Geometry: final body of the model. Coordinates: model frame, mm. A direction names the side the tool comes from. Coordinates: 2 decimals unless noted, no trailing zeros. Order: outer loops, then holes, each group sorted by start corner. A loop starts at its lowest first (then second) coordinate and runs counter-clockwise, first axis right, second up. Notation, with made-up numbers: (34, -12.5) -> (72, -12.5) arc R19 cw to (72, 19.5) -> close; hole circle Ø2 at (1, 13). An arc over 180 degrees is marked (long way). Answer in a Markdown table with one row per item. Add a question column.
1) Ray query, line 1 (Y direction, x = -2.75, z = 8); line 2 (Y direction, x = 8.25, z = 14.5); line 3 (Z direction, x = -5.75, y = 4). Return the intervals inside material, ascending. Write a range as from..to.
2) Set-up query: faces 1 (the face through (0, 2, 9.431)), 2 (the face through (-0.7, 2.1, 11.831)), 3 (the face through (6.972, 6.529, 14.967)), 4 (the face through (-2, 2, -5.169)). Return all of +Z, -Z, +X, -X, +Y, -Y with unobstructed straight access to the full face (end or side cutting, diameter ignored); none if empty.
3) Section query D-D on y = 1.5. Return the cut outline in (x, z).
4) Section query A-A on x = -5. Return the cut outline in (y, z), then the cut area to 3 significant figures.
5) Section query C-C on x = -2.5. Return the cut outline in (y, z), then the cut area to 3 significant figures.
6) Contact query for flat-ended pins moving along their axis: P1, Ø6, axis at x = -4, y = -1, coming from the -Z side; P2, Ø4, axis at y = -9.48, z = -8.17, coming from the -X side; P3, Ø3, axis at x = -6, y = 1, coming from the +Z side. Output: stop coordinate, or through.
7) Section query B-B on z = 9. Return the cut outline in (x, y), then the cut area to 3 significant figures.
8) Pull-direction query (X, two-part tool) for faces 5 (the face through (-2.29, 0.57, 10.65)), 6 (the face through (6.972, 13.65, -1.186)), 7 (the face through (-10, 9, 3)); classes: +X half, -X half, draft (parallel to the pull), parting line (faces both ways), or undercut.
Autodesk Fusion 360 part; units mm, degrees
sketch "Sketch2" plane through (5, 0, 0) normal (1, 0, 0) x (0, 1, 0)
  line L0 (16.9637, 18.2844) -> (-13.0292, -11.7227) construction
  line L1 (-12.9363, 18.2856) -> (17.0619, -11.7162) construction
  circle A0 centre (13.5169, 14.8306) radius 1.6
  circle A1 centre (-9.4831, 14.8306) radius 1.6
  circle A2 centre (-9.4831, -8.1694) radius 1.6
  circle A3 centre (13.5169, -8.1694) radius 1.6
  circle A4 centre (-9.4831, 14.8306) radius 4.1
  circle A5 centre (13.5169, 14.8306) radius 4.1
  circle A6 centre (-9.4831, -8.1694) radius 4.1
  line L2 (9.4619, 10.7862) -> (-5.5274, -4.2245) construction
  line L3 (-7.1431, 18.1972) -> (2.0169, 11.8306)
  line L4 (2.0169, 11.8306) -> (11.1769, 18.1972)
  line L5 (-12.8477, 12.4876) -> (-6.471, 3.3306)
  line L6 (-6.471, 3.3306) -> (-12.8477, -5.8265)
  line L7 (-7.1431, -11.5361) -> (2.0169, -5.1694)
  line L8 (10.5048, 3.3306) -> (16.8815, 12.4876)
  circle A7 centre (13.5169, -8.1694) radius 4.1
  line L9 (10.5048, 3.3306) -> (16.8815, -5.8265)
  line L10 (2.0169, -5.1694) -> (11.1769, -11.5361)
  line L11 (-4.0831, -2.7694) -> (8.1169, -2.7694)
  line L12 (8.1169, -2.7694) -> (8.1169, 9.4306)
  line L13 (8.1169, 9.4306) -> (-4.0831, 9.4306)
  line L14 (-4.0831, 9.4306) -> (-4.0831, -2.7694)
  line L15 (-4.0831, -2.7694) -> (8.1169, 9.4306) construction
  line L16 (8.1169, -2.7694) -> (-4.0831, 9.4306) construction
  line L17 (10.5048, 11.8306) -> (-6.471, 11.8306)
  line L18 (-6.471, 11.8306) -> (-6.471, -5.1694)
  line L19 (-6.471, -5.1694) -> (10.5048, -5.1694)
  line L20 (10.5048, -5.1694) -> (10.5048, 11.8306)
  line L21 (10.5048, 11.8306) -> (-6.471, -5.1694) construction
  line L22 (-6.471, 11.8306) -> (10.5048, -5.1694) construction
  point P0 (2.0169, 3.3306)
  point P1 (2.0169, 3.3306)
  point P2 (2.0169, 3.3306)
  point P3 (2.0169, 3.3306)
  point P4 (2.0169, 3.3306)
  dimension "d11" = 3.2
  dimension "d12" = 11.5
  dimension "d13" = 3.2
  dimension "d14" = 3.2
  dimension "d15" = 3.2
  dimension "d18" = 11.5
  dimension "d19" = 23
  dimension "d20" = 8.2
  dimension "d21" = 8.2
  dimension "d22" = 8.2
  dimension "d23" = 8.2
  dimension "d33" = 12.2
  dimension "d34" = 17
  dimension "d35" = 23
extrude "Extrude14" add sketch "Sketch2" along normal blind 5
extrude "Extrude16" add sketch "Sketch2" against normal blind 15 contours L17 L18 L19 L20
sketch "Sketch5" plane through (0, 0, 11.8306) normal (0, 0, 1) x (-1, 0, 0)
  line L0 (-5, -2.0169) -> (-5, -10.5048)
  line L1 (-5, -10.5048) -> (10, -10.5048)
  line L2 (10, -10.5048) -> (10, 6.471)
  line L3 (10, 6.471) -> (-5, 6.471)
  line L4 (-5, 6.471) -> (-5, -2.0169)
  circle A0 centre (2.5, -2.1573) radius 1.6
  circle A1 centre (2.5, -2.1573) radius 3.1
  dimension "d61" = 3.2
  dimension "d64" = 6.2
extrude "Extrude17" cut sketch "Sketch5" against normal blind 5 contours A0
move_face "MoveFace1" by (-1, 0, 0) 1 faces at (10, -3.3164, 12.0306)
extrude "Extrude18" [suppressed]
extrude "Extrude15" [suppressed]
extrude "Extrude3" [suppressed]
equation "d11 = motorScrewHole"
equation "d12 = boltDistance / 2"
equation "d13 = motorScrewHole"
equation "d14 = motorScrewHole"
equation "d15 = motorScrewHole"
equation "motorScrewHole = 3.2 mm"
equation "d18 = boltDistance / 2"
equation "d19 = boltDistance"
equation "d20 = motorScrewHole + 5 mm"
equation "d21 = motorScrewHole + 5 mm"
equation "d22 = motorScrewHole + 5 mm"
equation "d23 = motorScrewHole + 5 mm"
equation "d35 = boltDistance"
equation "boltDistance = 23 mm"
Result:
| question | item | result |
|---|---|---|
| 1 | line 1 | -6.47..-4.08, 8.12..10.5 |
| 1 | line 2 | -13.57..-11.05, -7.92..-1.82, 5.86..11.95, 15.08..17.6 |
| 1 | line 3 | -5.17..-2.77, 9.43..11.83 |
| 2 | face 1 | +X, -X |
| 2 | face 2 | +Z, -X, +Y, -Y |
| 2 | face 3 | +Z, +X, -X |
| 2 | face 4 | -Z, -X, +Y, -Y |
| 3 | outline | (-10, -5.17) -> (5, -5.17) -> (5, -5.53) -> (9, -5.53) -> (9, -2.77) -> (-10, -2.77) -> close; (-10, 9.43) -> (-3.96, 9.43) -> (-3.96, 11.83) -> (-10, 11.83) -> close; (-1.04, 9.43) -> (9, 9.43) -> (9, 12.19) -> (5, 12.19) -> (5, 11.83) -> (-1.04, 11.83) -> close |
| 4 | outline | (-6.47, -5.17) -> (10.5, -5.17) -> (10.5, 11.83) -> (-6.47, 11.83) -> close; hole (-4.08, -2.77) -> (8.12, -2.77) -> (8.12, 9.43) -> (-4.08, 9.43) -> close |
| 4 | area | 140 mm2 |
| 5 | outline | (-6.47, -5.17) -> (10.5, -5.17) -> (10.5, 11.83) -> (3.76, 11.83) -> (3.76, 9.43) -> (8.12, 9.43) -> (8.12, -2.77) -> (-4.08, -2.77) -> (-4.08, 9.43) -> (0.56, 9.43) -> (0.56, 11.83) -> (-6.47, 11.83) -> close |
| 5 | area | 132 mm2 |
| 6 | P1 | z = -5.17 |
| 6 | P2 | x = 5 |
| 6 | P3 | z = 11.83 |
| 7 | outline | (-10, -6.47) -> (5, -6.47) -> (5, -10.42) -> (9, -10.42) -> (9, -4.08) -> (-10, -4.08) -> close; (-10, 8.12) -> (9, 8.12) -> (9, 14.45) -> (5, 14.45) -> (5, 10.5) -> (-10, 10.5) -> close |
| 7 | area | 122 mm2 |
| 8 | face 5 | undercut |
| 8 | face 6 | draft |
| 8 | face 7 | -X half |
